from build123d import *

# Parameters (mm, degrees)
SKETCH1_R           = 4.845
SKETCH1_R_2         = 2.375
BOSS_EXTRUDE1_DEPTH = 5.75
SKETCH4_R           = 6.25
SKETCH4_R_2         = 2.375
BOSS_EXTRUDE4_DEPTH = 1
SKETCH5_R           = 4.845
SKETCH5_R_2         = 2.375
BOSS_EXTRUDE5_DEPTH = 5.75
SKETCH6_R           = 4.845
BOSS_EXTRUDE6_DEPTH = 2
SKETCH7_R           = 2.375
BOSS_EXTRUDE7_DEPTH = 50


with BuildPart() as part:
    # Sketch1 → Boss-Extrude1 (new body)
    with BuildSketch(Plane(origin=(0, 0, 0), x_dir=(1, 0, 0), z_dir=(0, 1, 0))):
        with Locations(Location((0, 0, 0), (0, 0, 270))):
            Circle(SKETCH1_R)
        with Locations(Location((0, 0, 0), (0, 0, 270))):
            Circle(SKETCH1_R_2, mode=Mode.SUBTRACT)
    extrude(amount=BOSS_EXTRUDE1_DEPTH)

    # Sketch4 → Boss-Extrude4 (add)
    with BuildSketch(Plane(origin=(0, 5.75, 0), x_dir=(1, 0, 0), z_dir=(0, 1, 0))):
        with Locations(Location((0, 0, 0), (0, 0, 270))):
            Circle(SKETCH4_R)
        with Locations(Location((0, 0, 0), (0, 0, 270))):
            Circle(SKETCH4_R_2, mode=Mode.SUBTRACT)
    extrude(amount=BOSS_EXTRUDE4_DEPTH)

    # Sketch5 → Boss-Extrude5 (add)
    with BuildSketch(Plane(origin=(0, 6.75, 0), x_dir=(1, 0, 0), z_dir=(0, 1, 0))):
        with Locations(Location((0, 0, 0), (0, 0, 270))):
            Circle(SKETCH5_R)
        with Locations(Location((0, 0, 0), (0, 0, 270))):
            Circle(SKETCH5_R_2, mode=Mode.SUBTRACT)
    extrude(amount=BOSS_EXTRUDE5_DEPTH)

    # Sketch6 → Boss-Extrude6 (add)
    with BuildSketch(Plane(origin=(0, 12.5, 0), x_dir=(1, 0, 0), z_dir=(0, 1, 0))):
        with Locations(Location((0, 0, 0), (0, 0, 270))):
            Circle(SKETCH6_R)
    extrude(amount=BOSS_EXTRUDE6_DEPTH)

    # Sketch7 → Boss-Extrude7 (add)
    with BuildSketch(Plane(origin=(0, 14.5, 0), x_dir=(1, 0, 0), z_dir=(0, 1, 0))):
        with Locations(Location((0, 0, 0), (0, 0, 270))):
            Circle(SKETCH7_R)
    extrude(amount=BOSS_EXTRUDE7_DEPTH)


solid = part.part
Design review of the part built by this model. Coordinates are the model's own, in mm. A direction names the side the tool comes from. Round coordinates to 2 decimals unless told otherwise and drop trailing zeros. Order: outer loops, then holes, each group sorted by start corner. A loop starts at its lowest first (then second) coordinate and runs counter-clockwise, first axis right, second up. Notation, with made-up numbers: M -4,71 L 45,71 A10 ccw 45,87 Z; hole C 17.5,-5.75 d9. An arc over 180 degrees is marked long. Answer as CSV lines item,"result". Start each with the question number.
1) Add section A-A (z = 0). Give the boundary of the cut face in (x, y) (3 decimals), then the cut area to 3 significant figures.
2) Add section B-B (x = 0). Give the boundary of the cut face in (y, z) (3 decimals).
3) Wall thickness on line 1 along X through (y, z) = (2.5, 0) (3 decimals); line 2 along Y through (x, z) = (-3.75, -2.75); line 3 along Y through (x, z) = (5.25, -0.25): over which ranges is each line inside the solid? List them lowest first. Write a range as [from, to].
4) Add section D-D (y = 48). Give the boundary of the cut face in (x, z) (3 decimals).
5) For pin 1 Ø5 at (x, y) = (1, 38.5) entering from +Z (3 decimals); pin 2 Ø4 at (x, y) = (-3.5, 57) entering from -Z; pin 3 Ø3 at (y, z) = (25.5, -3.5) entering from +X, all flat-tipped, find the tip position at first contact; note any pin that passes through.
6) Add section C-C (y = 4). Give the boundary of the cut face in (x, z) (3 decimals).
7) Tool access review of faces 4 (the face through (-1.45, 39.15, -1.88)), 5 (the face through (1.88, 6.24, 5.96)), 6 (the face through (0, 12.5, 0)): name each direction out of +Z, -Z, +X, -X, +Y, -Y from which nothing blocks a thin tool from reaching the whole face with its end or side.
8) The part is to be moulded in two halves that separate along Z. For faces 1 (the face through (-4, 5.75, 3)), 2 (the face through (4.804, 2.835, -0.631)), 3 (the face through (-1.45, 6.16, -1.88)), say which applies: +Z half, -Z half, draft (parallel to the pull), parting line (faces both ways), or undercut.
Resolved:
1,outline,"M -6.25,5.75 L -4.845,5.75 L -4.845,0 L -2.375,0 L -2.375,12.5 L 2.375,12.5 L 2.375,0 L 4.845,0 L 4.845,5.75 L 6.25,5.75 L 6.25,6.75 L 4.845,6.75 L 4.845,14.5 L 2.375,14.5 L 2.375,64.5 L -2.375,64.5 L -2.375,14.5 L -4.845,14.5 L -4.845,6.75 L -6.25,6.75 Z"
1,area,"321 mm^2"
2,outline,"M 0,-4.845 L 5.75,-4.845 L 5.75,-6.25 L 6.75,-6.25 L 6.75,-4.845 L 14.5,-4.845 L 14.5,-2.375 L 64.5,-2.375 L 64.5,2.375 L 14.5,2.375 L 14.5,4.845 L 6.75,4.845 L 6.75,6.25 L 5.75,6.25 L 5.75,4.845 L 0,4.845 L 0,2.375 L 12.5,2.375 L 12.5,-2.375 L 0,-2.375 Z"
3,line 1,"[-4.845, -2.375], [2.375, 4.845]"
3,line 2,"[0, 14.5]"
3,line 3,"[5.75, 6.75]"
4,outline,"C 0,0 d4.75"
5,pin 1,"z = 2.375"
5,pin 2,"z = -1.84"
5,pin 3,"x = 1.28"
6,outline,"C 0,0 d9.69; hole C 0,0 d4.75"
7,face 4,"+Y"
7,face 5,"+Y, -Y"
7,face 6,"-Y"
8,face 1,"draft"
8,face 2,"parting line"
8,face 3,"undercut"
